Input: part model. Units: mm. Frame: model coordinates. A direction names the side the tool comes from. Give positions to 0.01 mm unless a question says otherwise; leave off trailing zeros. Loops run counter-clockwise (first coordinate to the right, second up) from the corner with the lowest first, then second, coordinate; pieces in that order, holes last. Notation, with made-up numbers: (80, 52.5) - (96, 52.5) arc R16 ccw to (96, 79.5) - close; hole circle Ø6 at (47.5, 77). An arc over 180 degrees is marked (long way). One line per item, written item: value.
from build123d import *

# Parameters (mm, degrees)
SKETCH1_W           = 70.612
SKETCH1_H           = 29.718
BOSS_EXTRUDE1_DEPTH = 5.842
CUT_EXTRUDE1_DEPTH  = 6.842
CUT_EXTRUDE2_DEPTH  = 6.8420001


with BuildPart() as part:
    # Sketch1 → Boss-Extrude1 (new body)
    with BuildSketch(Plane(origin=(0, 0, 0), x_dir=(1, 0, 0), z_dir=(0, 1, 0))):
        Rectangle(SKETCH1_W, SKETCH1_H)
    extrude(amount=BOSS_EXTRUDE1_DEPTH)

    # Sketch2 → Cut-Extrude1 (cut, through all)
    with BuildSketch(Plane(origin=(0, 5.842, 0), x_dir=(1, 0, 0), z_dir=(0, 1, 0))):
        with BuildLine():
            Line((0.727778591, 7.239), (28.194, 7.239))
            add(Edge.make_bspline(
                [(28.194, -7.239), (30.226, 0), (28.194, 7.239)],
                knots=[0, 0, 0, 1, 1, 1], degree=2))
            Line((28.194, -7.239), (0.727778591, -7.239))
            add(Edge.make_bspline(
                [(0.727778591, -7.239), (-1.304221409, 0), (0.727778591, 7.239)],
                knots=[0, 0, 0, 1, 1, 1], degree=2))
        make_face()
    extrude(amount=-CUT_EXTRUDE1_DEPTH, mode=Mode.SUBTRACT)

    # Sketch3 → Cut-Extrude2 (cut, through all)
    with BuildSketch(Plane.XZ):
        with BuildLine():
            Line((-24.765, 4.191), (-15.367, 4.191))
            ThreePointArc((-15.367, 4.191), (-11.176, 0), (-15.367, -4.191))
            Line((-15.367, -4.191), (-24.765, -4.191))
            ThreePointArc((-24.765, -4.191), (-28.956, 0), (-24.765, 4.191))
        make_face()
    extrude(amount=-CUT_EXTRUDE2_DEPTH, mode=Mode.SUBTRACT)


solid = part.part
Item 1: Access query for faces 5 (the face through (-0.5, 5.842, -0.2)), 6 (the face through (15, 3, 7.239)). Directions: +Z, -Z, +X, -X, +Y, -Y. A direction counts if a zero-diameter tool reaches every point of the face in a straight line with its end or side. Return the directions, or none.
Verdict:
face 5: +Z, -Z, +X, -X, +Y
face 6: +Y, -Y
Item 2: Section B-B, the plane y = 1.25. Count the separate pieces of the cut face and the enclosed holes in it, and give its area (3 significant figures).
Verdict:
separate pieces: 1
enclosed holes: 2
area: 1,550 mm^2
Item 3: Section A-A, the plane x = 10.5. Output: boundary loops of the cut face in (y, z), and give its area (3 significant figures).
Verdict:
outline: (0, -14.86) - (5.84, -14.86) - (5.84, -7.24) - (0, -7.24) - close; (0, 7.24) - (5.84, 7.24) - (5.84, 14.86) - (0, 14.86) - close
area: 89.0 mm^2
Item 4: Draft query along X for faces 1 (the face through (35.306, 3, 0)), 2 (the face through (-11.177, 2.88, 0.092)), 3 (the face through (-28.955, 2.88, -0.092)), 4 (the face through (0, 3, -14.859)). Return one class per face: pulls with the +X half, pulls with the -X half, needs draft (parallel to the pull), parting line crosses it, or undercut.
Verdict:
face 1: pulls with the +X half
face 2: undercut
face 3: undercut
face 4: needs draft
Item 5: Material intervals for L1, parallel to Z at x = 25, y = 2.75; L2, parallel to Z at x = -24, y = 1.85; L3, parallel to X at y = 4.65, z = -2.5, sorted ascending.
Verdict:
L1: z = -14.86 to -7.24, 7.24 to 14.86
L2: z = -14.86 to -4.19, 4.19 to 14.86
L3: x = -35.31 to -28.13, -12 to -0.17, 29.09 to 35.31
